Source: three-view drawing plus pictorial views. Frame: mm from the lowest corner of the part. Coordinates: 2 decimals unless noted, no trailing zeros. Loops run counter-clockwise (first coordinate to the right, second up) from the corner with the lowest first, then second, coordinate; pieces in that order, holes last. Notation, with made-up numbers: (-8.75, -34) - (15.25, -34) arc R20 cw to (15.25, -18) - close; hole circle Ø5 at (3, -6). An arc over 180 degrees is marked (long way). Return JSON: item names as keys, results as strings.
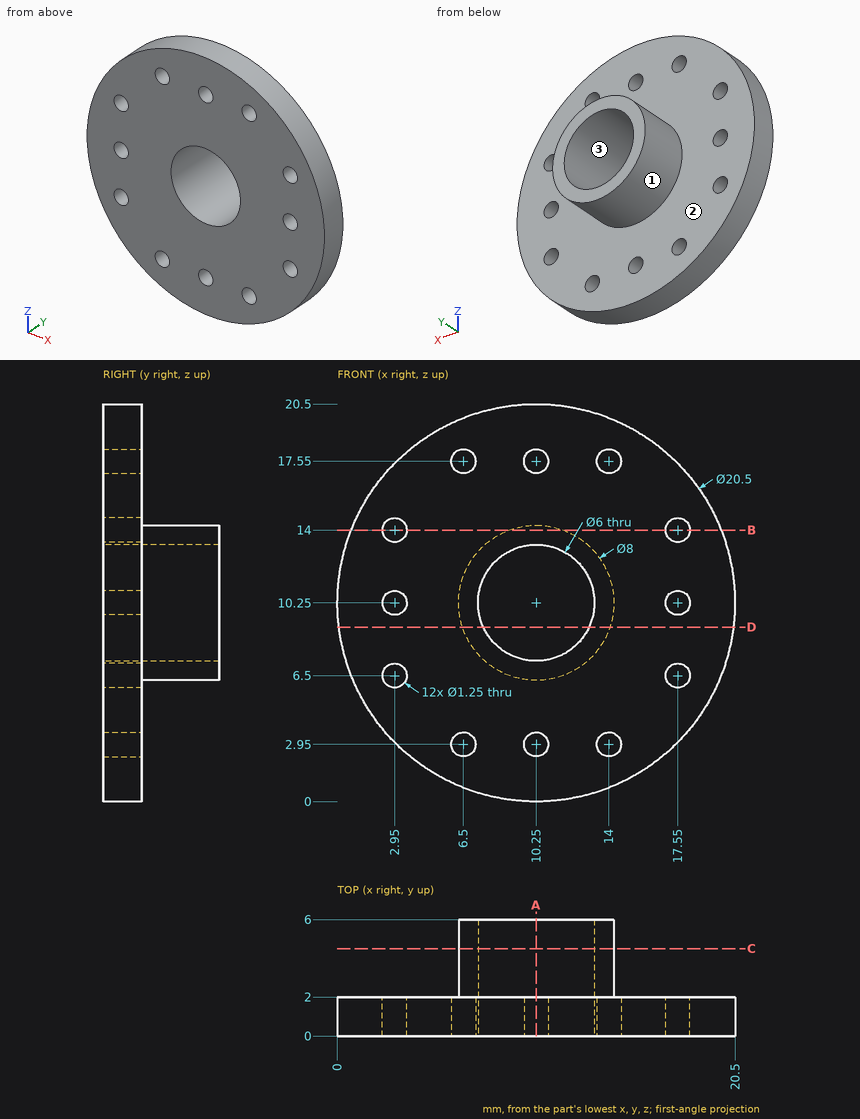
Item 1: Mould query, pull axis X, two halves, no side actions, for the marked faces 1, 2 and 3. Classes: +X half, -X half, draft (parallel to the pull), parting line (faces both ways), or undercut.
Worked out:
{"face 1": "parting line", "face 2": "draft", "face 3": "undercut"}
Item 2: Section query A-A, the plane x = 10.25. Return loops of the section in (y, z) (3 decimals), and give its area (3 significant figures).
Worked out:
{"outline": "(0, 0) - (2, 0) - (2, 2.325) - (0, 2.325) - close; (0, 3.575) - (2, 3.575) - (2, 6.25) - (6, 6.25) - (6, 7.25) - (0, 7.25) - close; (0, 13.25) - (6, 13.25) - (6, 14.25) - (2, 14.25) - (2, 16.925) - (0, 16.925) - close; (0, 18.175) - (2, 18.175) - (2, 20.5) - (0, 20.5) - close", "area": "32.0 mm^2"}
Item 3: Ray query, probe 1 along Z at (x, y) = (17.55, 0.45) (3 decimals); probe 2 along Z at (x, y) = (6.5, 0.9) (3 decimals); probe 3 along X at (y, z) = (2.4, 10.25). Return the intervals inside material, ascending. Write a range as from..to.
Worked out:
{"probe 1": "3.055..5.875, 7.125..9.625, 10.875..13.375, 14.625..17.445", "probe 2": "0.711..2.325, 3.575..16.925, 18.175..19.789", "probe 3": "6.25..7.25, 13.25..14.25"}
Item 4: First-contact query: pin 1 Ø1.1 at (x, z) = (2.95, 6.5) entering from -Y; pin 2 Ø1.6 at (x, z) = (14, 17.55) entering from +Y; pin 3 Ø3 at (y, z) = (1.5, 17) entering from -X; pin 4 Ø1 at (y, z) = (1.5, 17.5) entering from +X. Flat tips, straight axial feed; report the tip coordinate or a pass-through.
Worked out:
{"pin 1": "through", "pin 2": "y = 2", "pin 3": "x = 1.45", "pin 4": "x = 17.96"}
Item 5: Section query D-D, the plane z = 9. Return loops of the section in (x, y).
Worked out:
{"outline": "(0.08, 0) - (7.52, 0) - (7.52, 6) - (6.45, 6) - (6.45, 2) - (0.08, 2) - close; (12.98, 0) - (20.42, 0) - (20.42, 2) - (14.05, 2) - (14.05, 6) - (12.98, 6) - close"}
Item 6: Section query C-C, the plane y = 4.5. Return loops of the section in (x, z), and give its area (3 significant figures).
Worked out:
{"outline": "circle Ø8 at (10.25, 10.25); hole circle Ø6 at (10.25, 10.25)", "area": "22.0 mm^2"}
Item 7: Section query B-B, the plane z = 14. Return loops of the section in (x, y) (3 decimals), and give its area (3 significant figures).
Worked out:
{"outline": "(0.711, 0) - (2.325, 0) - (2.325, 2) - (0.711, 2) - close; (3.575, 0) - (16.925, 0) - (16.925, 2) - (11.642, 2) - (11.642, 6) - (8.858, 6) - (8.858, 2) - (3.575, 2) - close; (18.175, 0) - (19.789, 0) - (19.789, 2) - (18.175, 2) - close", "area": "44.3 mm^2"}
